from build123d import *

# Parameters (mm, degrees)
PAD_DEPTH       = 30
SKETCH001_R     = 2.3
POCKET_DEPTH    = 36.001
SKETCH002_R     = 2.2
POCKET001_DEPTH = 25.001


with BuildPart() as part:
    # Sketch → Pad (new body)
    with BuildSketch(Plane.XY):
        Polygon((27.992845, 15.579944), (-22.007155, 15.579944), (-22.007155, 10.579944), (-8.007155, 10.579944), (-8.007155, -9.420056), (-3.007155, -9.420056), (-3.007155, 10.579944), (8.992845, 10.579944), (8.992845, -9.420056), (13.992845, -9.420056), (13.992845, 10.579944), (27.992845, 10.579944), align=None)
    extrude(amount=PAD_DEPTH)

    # Sketch001 → Pocket (cut, through all)
    with BuildSketch(Plane.YZ.offset(13.992845)):
        with Locations((-1.920056, 7)):
            Circle(SKETCH001_R)
        with Locations((-1.920056, 23)):
            Circle(SKETCH001_R)
    extrude(amount=-POCKET_DEPTH, mode=Mode.SUBTRACT)

    # Sketch002 → Pocket001 (cut, through all)
    with BuildSketch(Plane(origin=(0, 15.579944, 0), x_dir=(-1, 0, 0), z_dir=(0, 1, 0))):
        with Locations((-22.992845, 7)):
            Circle(SKETCH002_R)
        with Locations((17.007155, 7)):
            Circle(SKETCH002_R)
        with Locations((-22.992845, 23)):
            Circle(SKETCH002_R)
        with Locations((17.007155, 23)):
            Circle(SKETCH002_R)
    extrude(amount=-POCKET001_DEPTH, mode=Mode.SUBTRACT)


solid = part.part
For this review, take the finished solid that the model builds, in its own axes (mm). A direction names the side the tool comes from. Give positions to 0.01 mm unless a question says otherwise; leave off trailing zeros. Loops run counter-clockwise (first coordinate to the right, second up) from the corner with the lowest first, then second, coordinate; pieces in that order, holes last. Notation, with made-up numbers: M 56,45 L 91,45 A22 cw 91,54 Z; hole C 80.25,66.5 d5. An arc over 180 degrees is marked long. Answer as a JSON object with one key per item and string values. Group by question number.
Q1. Insertion check: P1, Ø8, axis at x = 20.5, z = 14.5, coming from the -Y side; P2, Ø3, axis at y = -2, z = 10, coming from the +X side; P3, Ø1.5, axis at y = -5.5, z = 17.5, coming from the -X side; P4, Ø4, axis at y = -1.92, z = 7, coming from the -X side. Each pin has a flat end and moves straight along its axis. Give the tip position at first contact, or say it passes through.
Q2. Mouldability with a two-part tool opening along Y and no side actions: class faces 4 (the flat face through (-15, 10.58, 15)), 5 (the cylindrical face through (11.53, -0.86, 20.96)), 6 (the flat face through (-8.007, 1, 15)), 7 (the flat face through (3, 15.58, 15)) as +Y half, -Y half, draft (parallel to the pull), parting line (faces both ways), or undercut.
Q3. Tool access review of faces 1 (the flat face through (-3.007, 0, 15)), 2 (the flat face through (-6, -9.42, 15)), 3 (the flat face through (13.993, 0, 15)): name each direction out of +Z, -Z, +X, -X, +Y, -Y from which nothing blocks a thin tool from reaching the whole face with its end or side.
Q4. Add section A-A on y = 3.5. Give the boundary of the cut face in (x, z), and give its area (3 significant figures).
Q5. For probe 1 along X at (y, z) = (0, 16.25); probe 2 along Y at (x, z) = (-17.5, 16.25); probe 3 along Y at (x, z) = (-6.5, 8.75), list the stretches that pass through material, from the lowest coordinate up. Write a range as [from, to].
Q6. Add section D-D on x = 2. Give the boundary of the cut face in (y, z).
Q7. Add section B-B on z = 7. Give the boundary of the cut face in (x, y).
Q8. Add section C-C on z = 2.5. Give the boundary of the cut face in (x, y).
Checked values:
{
 "1": {"P1": "y = 10.58", "P2": "x = 13.99", "P3": "x = -8.01", "P4": "through"},
 "2": {"face 4": "-Y half", "face 5": "undercut", "face 6": "draft", "face 7": "+Y half"},
 "3": {"face 1": "+Z, -Z, -Y", "face 2": "+Z, -Z, +X, -X, -Y", "face 3": "+Z, -Z, +X, -Y"},
 "4": {"outline": "M -8.01,0 L -3.01,0 L -3.01,30 L -8.01,30 Z; M 8.99,0 L 13.99,0 L 13.99,30 L 8.99,30 Z", "area": "300 mm²"},
 "5": {"probe 1": "[-8.01, -3.01], [8.99, 13.99]", "probe 2": "[10.58, 15.58]", "probe 3": "[-9.42, -3.41], [-0.43, 15.58]"},
 "6": {"outline": "M 10.58,0 L 15.58,0 L 15.58,30 L 10.58,30 Z"},
 "7": {"outline": "M -22.01,10.58 L -19.21,10.58 L -19.21,15.58 L -22.01,15.58 Z; M -14.81,10.58 L -8.01,10.58 L -8.01,0.38 L -3.01,0.38 L -3.01,10.58 L 8.99,10.58 L 8.99,0.38 L 13.99,0.38 L 13.99,10.58 L 20.79,10.58 L 20.79,15.58 L -14.81,15.58 Z; M -8.01,-9.42 L -3.01,-9.42 L -3.01,-4.22 L -8.01,-4.22 Z; M 8.99,-9.42 L 13.99,-9.42 L 13.99,-4.22 L 8.99,-4.22 Z; M 25.19,10.58 L 27.99,10.58 L 27.99,15.58 L 25.19,15.58 Z"},
 "8": {"outline": "M -22.01,10.58 L -8.01,10.58 L -8.01,-9.42 L -3.01,-9.42 L -3.01,10.58 L 8.99,10.58 L 8.99,-9.42 L 13.99,-9.42 L 13.99,10.58 L 27.99,10.58 L 27.99,15.58 L -22.01,15.58 Z"}
}
